Here's how the part is built. I have some questions about the finished solid (model axes, mm). A direction names the side the tool comes from. Round coordinates to 2 decimals unless told otherwise and drop trailing zeros. Order: outer loops, then holes, each group sorted by start corner. A loop starts at its lowest first (then second) coordinate and runs counter-clockwise, first axis right, second up. Notation, with made-up numbers: (-33.75, 49.25) - (12.25, 49.25) arc R22 ccw to (12.25, 60.25) - close; hole circle Ø10 at (74.5, 47). An arc over 180 degrees is marked (long way). Answer as a JSON object with one key per item and string values.
```python
from build123d import *

# Parameters (mm, degrees)
F0_R     = 1.2192
F1_DEPTH = 0.8255
F2_W     = 5.969
F2_H     = 4.826
F2_W_2   = 5.461
F2_H_2   = 4.318
F3_DEPTH = 5.842
F2_R     = 0.254
F4_DEPTH = 0.508
F5_DEPTH = 5.08


with BuildPart() as f1:
    # F0 (on Top) → F1 (new body)
    with BuildSketch(Plane.XY):
        Polygon((4.2418, 0), (-4.2418, 0), (-4.2418, -7.8486), (-10.9982, -14.605), (-10.9982, -31.5214), (-2.9718, -39.1668), (-2.9718, -45.593), (2.9718, -45.593), (2.9718, -39.1668), (10.9982, -31.5214), (10.9982, -14.605), (4.2418, -7.8486), align=None)
        with Locations((-7.874, -23.0632)):
            Circle(F0_R, mode=Mode.SUBTRACT)
        with Locations((0, -40.8432)):
            Circle(F0_R, mode=Mode.SUBTRACT)
        with Locations((7.874, -23.0632)):
            Circle(F0_R, mode=Mode.SUBTRACT)
        with Locations((0, -12.7508)):
            Circle(F0_R, mode=Mode.SUBTRACT)
    extrude(amount=F1_DEPTH)

    # F2 (on face) → F3 (join)
    with BuildSketch(Plane.XY.offset(0.8255)):
        with Locations((0, -5.207)):
            Rectangle(F2_W, F2_H)
        with Locations((0, -5.207)):
            Rectangle(F2_W_2, F2_H_2, mode=Mode.SUBTRACT)
    extrude(amount=F3_DEPTH)

    # F2 (on face) → F4 (join)
    with BuildSketch(Plane.XY.offset(0.8255)):
        with Locations((0, -5.207)):
            Rectangle(F2_W_2, F2_H_2)
        with Locations((-1.27, -6.35)):
            Circle(F2_R, mode=Mode.SUBTRACT)
        with Locations((1.27, -6.35)):
            Circle(F2_R, mode=Mode.SUBTRACT)
    extrude(amount=F4_DEPTH)

    # F2 (on face) → F5 (join)
    with BuildSketch(Plane.XY.offset(0.8255)):
        with Locations((-1.27, -6.35)):
            Circle(F2_R)
        with Locations((1.27, -6.35)):
            Circle(F2_R)
    extrude(amount=F5_DEPTH)


solid = f1.part
```
1. Imagine slicing it at D-D (y = -21). List the corners of the cut face in (x, z) for me.
Responses:
{"outline": "(-11, 0) - (11, 0) - (11, 0.83) - (-11, 0.83) - close"}
2. Imagine slicing it at B-B (z = 4). List the corners of the cut face in (x, y) for me.
Responses:
{"outline": "(-2.98, -7.62) - (2.98, -7.62) - (2.98, -2.79) - (-2.98, -2.79) - close; circle Ø0.51 at (-1.27, -6.35); circle Ø0.51 at (1.27, -6.35); hole (-2.73, -7.37) - (2.73, -7.37) - (2.73, -3.05) - (-2.73, -3.05) - close"}
3. For faces 5 (the face through (0, -2.794, 4)), 6 (the face through (-2.984, -5, 4)), 7 (the face through (0, -7.366, 4)), which set-ups out of +Z, -Z, +X, -X, +Y, -Y let a thin tool reach every point of the face, with its end or its side?
Responses:
{"face 5": "+Z, +X, -X, +Y", "face 6": "+Z, -X, +Y, -Y", "face 7": "+Z"}
4. If I drill on L1, parallel to Y at x = 0, z = 0.4; L2, parallel to Y at x = 1.25, z = 6; L3, parallel to X at y = -6.5, z = 2, over which ranges is the centre line in solid material (lowest first)? Write a range as [from, to].
Responses:
{"L1": "[-45.59, -42.06], [-39.62, -13.97], [-11.53, 0]", "L2": "[-7.62, -7.37], [-3.05, -2.79]", "L3": "[-2.98, -2.73], [-1.47, -1.07], [1.07, 1.47], [2.73, 2.98]"}
5. For P1, Ø0.7, axis at y = -5.5, z = 0.5, coming from the +X side; P2, Ø1.5, axis at x = 2, z = 5, coming from the -Y side; P3, Ø1.4, axis at y = -5, z = 4, coming from the -X side, each with a flat end and sliding along its axis, tell me the tip position at first contact or that it passes through.
Responses:
{"P1": "x = 4.24", "P2": "y = -7.62", "P3": "x = -2.98"}
6. Imagine slicing it at A-A (x = 0). List the corners of the cut face in (y, z) for me, plus the area to 3 significant figures.
Responses:
{"outline": "(-45.59, 0) - (-42.06, 0) - (-42.06, 0.83) - (-45.59, 0.83) - close; (-39.62, 0) - (-13.97, 0) - (-13.97, 0.83) - (-39.62, 0.83) - close; (-11.53, 0) - (0, 0) - (0, 0.83) - (-2.79, 0.83) - (-2.79, 6.67) - (-3.05, 6.67) - (-3.05, 1.33) - (-7.37, 1.33) - (-7.37, 6.67) - (-7.62, 6.67) - (-7.62, 0.83) - (-11.53, 0.83) - close", "area": "38.8 mm2"}
7. Thinking about a two-plate mould opening in X: for faces 1 (the face through (-8.033, -21.854, 0.407)), 2 (the face through (0, -7.62, 4)), 3 (the face through (2.972, -42.4, 0.4)), 4 (the face through (-0.264, -42.033, 0.407)), which applies, pulls with the +X half, pulls with the -X half, needs draft (parallel to the pull), parting line crosses it, or undercut?
Responses:
{"face 1": "undercut", "face 2": "needs draft", "face 3": "pulls with the +X half", "face 4": "undercut"}
8. Imagine slicing it at C-C (x = 8). List the corners of the cut face in (y, z) for me.
Responses:
{"outline": "(-34.38, 0) - (-24.28, 0) - (-24.28, 0.83) - (-34.38, 0.83) - close; (-21.85, 0) - (-11.61, 0) - (-11.61, 0.83) - (-21.85, 0.83) - close"}
